```python
from build123d import *

# Parameters (mm, degrees)
SKETCH_1_R      = 5
EXTRUDE_1_DEPTH = 10


with BuildPart() as part:
    # 草图1 → 凸台-拉伸1 (new body)
    with BuildSketch(Plane(origin=(0, 0, 0), x_dir=(1, 0, 0), z_dir=(0, 1, 0))):
        with BuildLine():
            Line((-50, 0), (-50, 30))
            Line((-50, 30), (-30, 30))
            Line((-30, 30), (-30, 0))
            ThreePointArc((-30, 0), (21.213203436, -21.213203436), (0, 30))
            ThreePointArc((0, 30), (-10, 40), (0, 50))
            ThreePointArc((0, 50), (35.355339059, -35.355339059), (-50, 0))
        make_face()
        with Locations(Location((0, 40, 0), (0, 0, 270))):
            Circle(SKETCH_1_R, mode=Mode.SUBTRACT)
    extrude(amount=EXTRUDE_1_DEPTH)


solid = part.part
```
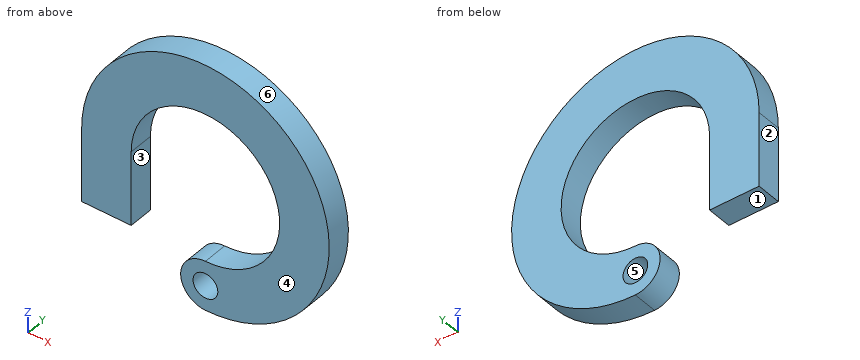
Design review of the part built by this model. Coordinates are the model's own, in mm. Face numbers are marked on the shaded views. A direction names the side the tool comes from. Give positions to 0.01 mm unless a question says otherwise; leave off trailing zeros. Order: outer loops, then holes, each group sorted by start corner. A loop starts at its lowest first (then second) coordinate and runs counter-clockwise, first axis right, second up. Notation, with made-up numbers: (80, -16) -> (92, -16) arc R25 ccw to (92, 7) -> close; hole circle Ø4 at (81.25, -26.5). An arc over 180 degrees is marked (long way). Write item = value, one per line. Start each with the question number.
(1) For pin 1 (3 mm diameter, centred on y = 5, z = -21, fed in from +X); pin 2 (6 mm diameter, centred on x = 5, y = 8, fed in from -Z); pin 3 (1.5 mm diameter, centred on y = 2, z = -32.5, fed in from +X), all flat-tipped, find the tip position at first contact; note any pin that passes through.
(2) We need section D-D on z = 7. Write out the cut boundary in (x, y), plus the area to 3 significant figures.
(3) For the marked faces 1 and 2, list the 3-axis set-ups (+Z, -Z, +X, -X, +Y, -Y) from which the entire face can be reached by the end or side of a thin tool; tool diameter is ignored.
(4) We need section C-C on x = 40. Write out the cut boundary in (y, z), plus the area to 3 significant figures.
(5) To check wall thickness, follow line 1 along X through (y, z) = (5.25, -40); line 2 along Z through (x, y) = (-3, 8.75); line 3 along X through (y, z) = (3.25, -8). State the ranges of each line that lie inside material, in increasing order.
(6) We need section B-B on y = 4. Write out the cut boundary in (x, z).
(7) Mouldability with a two-part tool opening along X and no side actions: class the marked faces 3, 4, 5 and 6 as +X half, -X half, draft (parallel to the pull), parting line (faces both ways), or undercut.
(8) We need section A-A on z = -40. Write out the cut boundary in (x, y).
Numbers:
q1.pin_1 = 46.04
q1.pin_2 = -49.96
q1.pin_3 = 38.63
q2.outline = (-49.51, 0) -> (-29.17, 0) -> (-29.17, 10) -> (-49.51, 10) -> close; (29.17, 0) -> (49.51, 0) -> (49.51, 10) -> (29.17, 10) -> close
q2.area = 407 mm^2
q3.face_1 = -Z, -X, +Y, -Y
q3.face_2 = +Z, -Z, -X, +Y, -Y
q4.outline = (0, -30) -> (10, -30) -> (10, 30) -> (0, 30) -> close
q4.area = 600 mm^2
q5.line_1 = -10 to -5, 5 to 30
q5.line_2 = -49.54 to -44, -36 to -30.46, 29.85 to 49.91
q5.line_3 = -50 to -30, 28.91 to 49.36
q6.outline = (-50, -30) -> (-30, -30) -> (-30, 0) arc R30 cw (long way) to (0, -30) arc R10 ccw to (0, -50) arc R50 ccw (long way) to (-50, 0) -> close; hole circle Ø10 at (0, -40)
q7.face_3 = undercut
q7.face_4 = draft
q7.face_5 = undercut
q7.face_6 = parting line
q8.outline = (-10, 0) -> (-5, 0) -> (-5, 10) -> (-10, 10) -> close; (5, 0) -> (30, 0) -> (30, 10) -> (5, 10) -> close
